Can you work these out from the model? Positions are in its coordinate system, mm. A direction names the side the tool comes from. Round coordinates to 2 decimals unless told otherwise and drop trailing zeros. Write each loop counter-clockwise with the first axis right and the second up, starting at its lowest first coordinate (ties: lowest second). Pieces come first, ordered by that corner, then holes. Notation, with made-up numbers: M 68.5,0.5 L 124.5,0.5 A29 ccw 124.5,29.5 Z; hole C 69.5,7 d11. An arc over 180 degrees is marked long. Answer in a Markdown table with one row per item. Add a question column.
(1) Suppose I cut it at C-C, the plane x = 12.7. Write out the boundary of the cut face in (y, z).
(2) If I drill on probe 1 along Y at (x, z) = (12.7, 2.5); probe 2 along Y at (x, z) = (13, 10.75); probe 3 along Y at (x, z) = (57.15, 9), over which ranges is the centre line in solid material (lowest first)?
(3) Suppose I cut it at B-B, the plane x = 88.9. Write out the boundary of the cut face in (y, z), then the cut area to 3 significant figures.
(4) Suppose I cut it at D-D, the plane y = 8.5. Write out the boundary of the cut face in (x, z).
(5) For faces 4 (the face through (61, 24, 4.775)), 5 (the face through (47, 32, 0)), 6 (the face through (13.9, 48.55, 3.13)), which set-ups out of +Z, -Z, +X, -X, +Y, -Y let a thin tool reach every point of the face, with its end or its side?
(6) If we mould it in two halves opening along X, with no side actions, what happens to faces 1 (the face through (47, 63.5, 6)), 2 (the face through (73.28, 25.06, 8.79)), 3 (the face through (0, 31, 6))? For each: released by +X, released by -X, zero draft, split by the parting line, or undercut.
(7) I'm going to push flat-ended pins straight in: pin 1 (17.5 mm diameter, centred on x = 60, y = 33, fed in from +Z); pin 2 (3.5 mm diameter, centred on x = 12.5, y = 52, fed in from -Z). Where does each tip first touch, or does it pass through?
(8) Suppose I cut it at A-A, the plane y = 31.75. Write out the boundary of the cut face in (x, z), then the cut area to 3 significant figures.
from build123d import *

# Parameters (mm, degrees)
SKETCH1_W                                        = 95.25
SKETCH1_H                                        = 63.5
BOSS_EXTRUDE1_DEPTH                              = 12.7
CBORE_FOR_1_4_SOCKET_HEAD_CAP_SCREW1_D           = 7.14248
CBORE_FOR_1_4_SOCKET_HEAD_CAP_SCREW1_CBORE_D     = 11.1125
CBORE_FOR_1_4_SOCKET_HEAD_CAP_SCREW1_CBORE_DEPTH = 6.35
CBORE_FOR_5_8_SOCKET_HEAD_CAP_SCREW1_D           = 16.256
CBORE_FOR_5_8_SOCKET_HEAD_CAP_SCREW1_CBORE_D     = 34.925
CBORE_FOR_5_8_SOCKET_HEAD_CAP_SCREW1_CBORE_DEPTH = 7.9248
F_8_32_TAPPED_HOLE1_D                            = 3.4544


with BuildPart() as part:
    # Sketch1 → Boss-Extrude1 (new body)
    with BuildSketch(Plane.XY):
        with Locations((47.625, 31.75)):
            Rectangle(SKETCH1_W, SKETCH1_H)
    extrude(amount=BOSS_EXTRUDE1_DEPTH)

    # CBORE for 1/4 Socket Head Cap Screw1 (through all)
    with Locations(Plane(origin=(0, 0, 0), x_dir=(-1, 0, 0), z_dir=(0, 0, -1))):
        with Locations((-12.7, 53.975), (-12.7, 9.525)):
            CounterBoreHole(CBORE_FOR_1_4_SOCKET_HEAD_CAP_SCREW1_D / 2, CBORE_FOR_1_4_SOCKET_HEAD_CAP_SCREW1_CBORE_D / 2, CBORE_FOR_1_4_SOCKET_HEAD_CAP_SCREW1_CBORE_DEPTH)

    # CBORE for 5/8 Socket Head Cap Screw1 (through all)
    with Locations(Plane.XY.offset(12.7)):
        with Locations((57.15, 31.75)):
            CounterBoreHole(CBORE_FOR_5_8_SOCKET_HEAD_CAP_SCREW1_D / 2, CBORE_FOR_5_8_SOCKET_HEAD_CAP_SCREW1_CBORE_D / 2, CBORE_FOR_5_8_SOCKET_HEAD_CAP_SCREW1_CBORE_DEPTH)

    # #8-32 Tapped Hole1 (through all)
    with Locations(Plane.XY.offset(12.7)):
        with Locations((88.9, 31.75)):
            Hole(F_8_32_TAPPED_HOLE1_D / 2)


solid = part.part
Calculated:
| question | item | result |
|---|---|---|
| 1 | outline | M 0,0 L 3.97,0 L 3.97,6.35 L 5.95,6.35 L 5.95,12.7 L 0,12.7 Z; M 13.1,6.35 L 15.08,6.35 L 15.08,0 L 48.42,0 L 48.42,6.35 L 50.4,6.35 L 50.4,12.7 L 13.1,12.7 Z; M 57.55,6.35 L 59.53,6.35 L 59.53,0 L 63.5,0 L 63.5,12.7 L 57.55,12.7 Z |
| 2 | probe 1 | 0 to 3.97, 15.08 to 48.42, 59.53 to 63.5 |
| 2 | probe 2 | 0 to 5.97, 13.08 to 50.42, 57.53 to 63.5 |
| 2 | probe 3 | 0 to 14.29, 49.21 to 63.5 |
| 3 | outline | M 0,0 L 30.02,0 L 30.02,12.7 L 0,12.7 Z; M 33.48,0 L 63.5,0 L 63.5,12.7 L 33.48,12.7 Z |
| 3 | area | 763 mm² |
| 4 | outline | M 0,0 L 7.24,0 L 7.24,6.35 L 9.28,6.35 L 9.28,12.7 L 0,12.7 Z; M 16.12,6.35 L 18.16,6.35 L 18.16,0 L 95.25,0 L 95.25,12.7 L 16.12,12.7 Z |
| 5 | face 4 | +Z |
| 5 | face 5 | -Z, +X, -X, +Y, -Y |
| 5 | face 6 | -Z |
| 6 | face 1 | zero draft |
| 6 | face 2 | undercut |
| 6 | face 3 | released by -X |
| 7 | pin 1 | z = 4.78 |
| 7 | pin 2 | z = 6.35 |
| 8 | outline | M 0,0 L 49.02,0 L 49.02,4.78 L 39.69,4.78 L 39.69,12.7 L 0,12.7 Z; M 65.28,0 L 87.17,0 L 87.17,12.7 L 74.61,12.7 L 74.61,4.78 L 65.28,4.78 Z; M 90.63,0 L 95.25,0 L 95.25,12.7 L 90.63,12.7 Z |
| 8 | area | 811 mm² |
